Geometry check sheet. Reference: the model listing, model coordinates, mm. A direction names the side the tool comes from. Round coordinates to 2 decimals unless told otherwise and drop trailing zeros. Loops run counter-clockwise (first coordinate to the right, second up) from the corner with the lowest first, then second, coordinate; pieces in that order, holes last.
```python
from build123d import *

# Parameters (mm, degrees)
CHAMFER003_SIZE  = 0.25
CHAMFER004_SIZE2 = 0.5
CHAMFER004_SIZE  = 1


with BuildPart() as part:
    # Sketch007 → Revolution (revolve)
    with BuildSketch(Plane.XY):
        with BuildLine():
            Line((4, 18.375), (5.875, 18.375))
            Line((5.875, 18.375), (5.875, 17.375))
            ThreePointArc((5.875, 17.375), (4.7938611699, 15.875), (5.875, 14.375))
            Line((5.875, 14.375), (5.875, 7.125))
            Line((5.875, 7.125), (6.625, 7.125))
            Line((6.625, 3.625), (6.625, 7.125))
            Line((4, 3.625), (6.625, 3.625))
            Line((4, 18.375), (4, 3.625))
        make_face()
    revolve(axis=Axis((0, 0, 0), (0, 1, 0)))

    # Chamfer003
    chamfer003_edges = [part.edges().sort_by_distance(p)[0] for p in [
        (-4, 18.375, 0),
        (-5.875, 18.375, 0),
    ]]
    chamfer(chamfer003_edges, length=CHAMFER003_SIZE)

    # Chamfer004
    chamfer004_edges = [part.edges().sort_by_distance(p)[0] for p in [
        (-6.625, 3.625, 0),
    ]]
    chamfer004_side = part.faces().sort_by_distance((-4.187383, 3.625, 0))[0]
    chamfer(chamfer004_edges, length=CHAMFER004_SIZE, length2=CHAMFER004_SIZE2, reference=chamfer004_side)


with BuildPart() as part_1:
    # Body006 placement: moved
    add(part.part.moved(Location((12.5, 0, 0))))


solid = part_1.part
```
1) Sectioned sample at A-A, the plane z = 0. Record the cut outline in (x, y) (3 decimals).
Report:
outline: (5.875, 4.125) - (6.875, 3.625) - (8.5, 3.625) - (8.5, 18.125) - (8.25, 18.375) - (6.875, 18.375) - (6.625, 18.125) - (6.625, 17.375) arc R1.581 cw to (6.625, 14.375) - (6.625, 7.125) - (5.875, 7.125) - close; (16.5, 3.625) - (18.125, 3.625) - (19.125, 4.125) - (19.125, 7.125) - (18.375, 7.125) - (18.375, 14.375) arc R1.581 cw to (18.375, 17.375) - (18.375, 18.125) - (18.125, 18.375) - (16.75, 18.375) - (16.5, 18.125) - close
2) Sectioned sample at B-B, the plane x = 12.5. Record the cut outline in (y, z) (3 decimals).
Report:
outline: (3.625, -5.625) - (4.125, -6.625) - (7.125, -6.625) - (7.125, -5.875) - (14.375, -5.875) arc R1.581 cw to (17.375, -5.875) - (18.125, -5.875) - (18.375, -5.625) - (18.375, -4.25) - (18.125, -4) - (3.625, -4) - close; (3.625, 4) - (18.125, 4) - (18.375, 4.25) - (18.375, 5.625) - (18.125, 5.875) - (17.375, 5.875) arc R1.581 cw to (14.375, 5.875) - (7.125, 5.875) - (7.125, 6.625) - (4.125, 6.625) - (3.625, 5.625) - close
3) Gauge pin test, flat ends, axial feed: pin 1 (1.5 mm diameter, centred on x = 18, y = 6, fed in from +Z); pin 2 (5 mm diameter, centred on x = 12.5, z = 0, fed in from -Y); pin 3 (3 mm diameter, centred on x = 10.5, y = 10, fed in from +Z). Record the tip position at first contact, or that the pin passes through.
Report:
pin 1: stops at z = 4.62
pin 2: passes through
pin 3: stops at z = 5.85
4) Scan lines: line 1 along Z through (x, y) = (12.5, 7.5) (3 decimals); line 2 along X through (y, z) = (12.5, 0) (3 decimals); line 3 along Z through (x, y) = (12.5, 7) (3 decimals). Record each from-to range of solid material in increasing order.
Report:
line 1: z = -5.875 to -4, 4 to 5.875
line 2: x = 6.625 to 8.5, 16.5 to 18.375
line 3: z = -6.625 to -4, 4 to 6.625
5) Mould release check, pull along Z, two halves, no side actions. Record for faces 3 (the face through (9.3, 10.8, 2.4)), 4 (the face through (15, 18.375, -4)), 5 (the face through (18.82, 5.65, -1.99)): +Z half, -Z half, draft (parallel to the pull), parting line (faces both ways), or undercut.
Report:
face 3: undercut
face 4: draft
face 5: parting line
6) Sectioned sample at D-D, the plane y = 13. Record the cut outline in (x, z) (3 decimals), then the cut area to 3 significant figures.
Report:
outline: circle Ø11.75 at (12.5, 0); hole circle Ø8 at (12.5, 0)
area: 58.2 mm2
7) Sectioned sample at C-C, the plane y = 5.5. Record the cut outline in (x, z) (3 decimals).
Report:
outline: circle Ø13.25 at (12.5, 0); hole circle Ø8 at (12.5, 0)
8) Access from +Z, -Z, +X, -X, +Y, -Y to the whole of each face (thin tool, end or side, straight path). Record for faces 1 (the face through (14, 7.125, 6)), 2 (the face through (11, 3.625, -4)).
Report:
face 1: +Y
face 2: +Z, -Z, +X, -X, -Y
